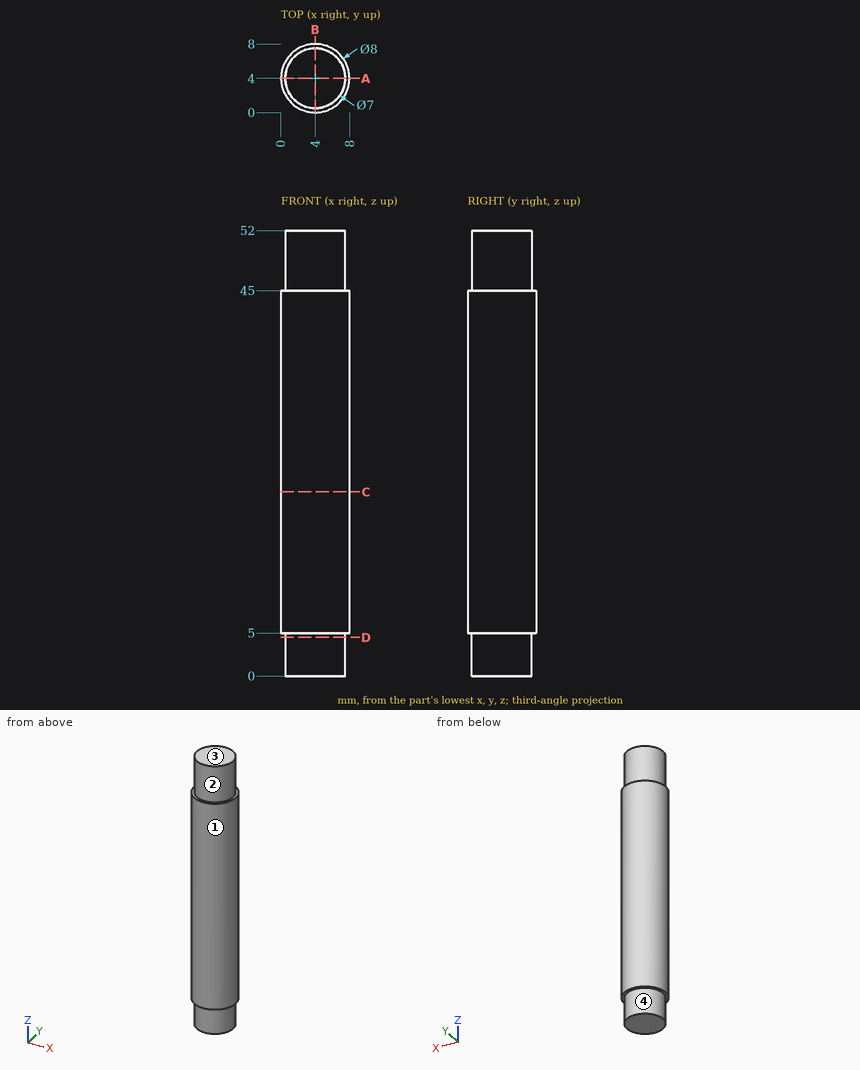
Part print with two shaded views. Sizes in mm from the minimum x, y, z corner. A direction names the side the tool comes from. Round coordinates to 2 decimals unless told otherwise and drop trailing zeros. Order: outer loops, then holes, each group sorted by start corner. A loop starts at its lowest first (then second) coordinate and runs counter-clockwise, first axis right, second up. Notation, with made-up numbers: (-15.75, 44.25) - (-10.75, 44.25) arc R36 cw to (-10.75, 79.25) - close; hole circle Ø2 at (66.5, 82). An arc over 180 degrees is marked (long way). Return JSON: item names as keys, results as strings.
(1) Cut at C-C (z = 21.5). Give the cut face in (x, y), then the cut area to 3 significant figures.
Answer key:
{"outline": "circle Ø8 at (4, 4)", "area": "50.3 mm^2"}
(2) Pull direction X, two halves, no side cores. Call the marked faces 3 and 4: +X half, -X half, draft (parallel to the pull), parting line (faces both ways), or undercut.
Answer key:
{"face 3": "draft", "face 4": "parting line"}
(3) Wall check: probe 1 along Z at (x, y) = (7.25, 5.75); probe 2 along X at (y, z) = (5, 41.5); probe 3 along X at (y, z) = (0.75, 12). Give the ranges that are in metal, low to high. Write a range as from..to.
Answer key:
{"probe 1": "z = 5..45", "probe 2": "x = 0.13..7.87", "probe 3": "x = 1.67..6.33"}
(4) Pin check, flat tips, straight feed: pin 1 Ø1.5 at (x, z) = (5, 42.5) entering from -Y; pin 2 Ø2 at (x, y) = (5, 6.5) entering from -Z; pin 3 Ø2 at (y, z) = (1, 11) entering from +X; pin 4 Ø4 at (x, z) = (7, 25.5) entering from -Y. Stop position of each tip, or through.
Answer key:
{"pin 1": "stops at y = 0.01", "pin 2": "stops at z = 0", "pin 3": "stops at x = 7.46", "pin 4": "stops at y = 0.13"}
(5) Cut at D-D (z = 4.5). Give the cut face in (x, y), then the cut area to 3 significant figures.
Answer key:
{"outline": "circle Ø7 at (4, 4)", "area": "38.5 mm^2"}
(6) Tool access for the marked faces 1 and 2: list every direction of +Z, -Z, +X, -X, +Y, -Y with a clear straight run to the whole face (end or side of a thin tool).
Answer key:
{"face 1": "+Z, -Z", "face 2": "+Z"}
(7) Cut at A-A (y = 4). Give the cut face in (x, z).
Answer key:
{"outline": "(0, 5) - (0.5, 5) - (0.5, 0) - (7.5, 0) - (7.5, 5) - (8, 5) - (8, 45) - (7.5, 45) - (7.5, 52) - (0.5, 52) - (0.5, 45) - (0, 45) - close"}
